from build123d import *

# Parameters (mm, degrees)
SKETCH1_R                = 85
BOSS_EXTRUDE1_DEPTH      = 3.175
SKETCH2_W                = 20
SKETCH2_H                = 18.160284919
SKETCH2_R                = 1.5
BOSS_EXTRUDE2_DEPTH      = 3.175
FILLET1_R                = 8
CIRPATTERN1_COUNT        = 3
FILLET1_OF_CIRPATTERN1_R = 8


with BuildPart() as part:
    # Sketch1 → Boss-Extrude1 (new body)
    with BuildSketch(Plane.XY):
        Circle(SKETCH1_R)
    extrude(amount=BOSS_EXTRUDE1_DEPTH)

    # Sketch2 → Boss-Extrude2 (add, through all)
    with BuildSketch(Plane.XY):
        with Locations((0, -93.48985754)):
            Rectangle(SKETCH2_W, SKETCH2_H)
        with Locations((0, -92.57)):
            Circle(SKETCH2_R, mode=Mode.SUBTRACT)
    boss_extrude2 = extrude(amount=BOSS_EXTRUDE2_DEPTH)

    # Fillet1
    fillet1_edges = [part.edges().sort_by_distance(p)[0] for p in [
        (-10, -84.409715081, 1.5875),
        (-10, -102.57, 1.5875),
        (10, -102.57, 1.5875),
        (10, -84.409715081, 1.5875),
    ]]
    fillet(fillet1_edges, radius=FILLET1_R)

    # CirPattern1: Boss-Extrude2 ×3 about axis
    cirpattern1_axis = Axis((0, 0, 0), (0, 0, 1))
    for i in range(1, CIRPATTERN1_COUNT):
        add(boss_extrude2.rotate(cirpattern1_axis, i * 360 / CIRPATTERN1_COUNT))

    # Fillet1 of CirPattern1
    fillet1_of_cirpattern1_edges = [part.edges().sort_by_distance(p)[0] for p in [
        (78.100957586, 33.544603502, 1.5875),
        (93.828225666, 42.624745962, 1.5875),
        (83.828225666, 59.945254038, 1.5875),
        (68.100957586, 50.865111578, 1.5875),
        (-68.100957586, 50.865111578, 1.5875),
        (-83.828225666, 59.945254038, 1.5875),
        (-93.828225666, 42.624745962, 1.5875),
        (-78.100957586, 33.544603502, 1.5875),
    ]]
    fillet(fillet1_of_cirpattern1_edges, radius=FILLET1_OF_CIRPATTERN1_R)


solid = part.part
Source: CAD feature listing. Evaluate the final solid. Frame: model axes, mm. Coordinates: 2 decimals unless noted, no trailing zeros. Loops run counter-clockwise (first coordinate to the right, second up) from the corner with the lowest first, then second, coordinate; pieces in that order, holes last. Notation, with made-up numbers: (-4.5, 15.5) - (12.5, 15.5) arc R22 cw to (12.5, 49.5) - close; hole circle Ø1 at (71.25, 19). An arc over 180 degrees is marked (long way). Return JSON: item names as keys, results as strings.
Q1. Contact query for flat-ended pins moving along their axis: P1, Ø1, axis at y = -92.5, z = 1.5, coming from the -X side; P2, Ø1.8, axis at x = 0, y = -92.57, coming from the -Z side. Output: stop coordinate, or through.
Results:
{"P1": "x = -10", "P2": "through"}
Q2. Material intervals for line 1 along Y through (x, z) = (0, 1.9); line 2 along X through (y, z) = (-92.57, 1.6); line 3 along X through (y, z) = (47, 2.8), sorted ascending.
Results:
{"line 1": "-102.57 to -94.07, -91.07 to 85", "line 2": "-10 to -1.5, 1.5 to 10", "line 3": "-90.77 to -81.49, -78.85 to 78.85, 81.49 to 90.77"}
Q3. Section C-C, the plane x = 53.5. Return loops of the section in (y, z) (3 decimals), plus the area to 3 significant figures.
Results:
{"outline": "(-66.051, 0) - (66.051, 0) - (66.051, 3.175) - (-66.051, 3.175) - close", "area": "419 mm2"}
Q4. Section B-B, the plane y = -17. Return loops of the section in (x, z) (3 decimals), plus the area to 3 significant figures.
Results:
{"outline": "(-83.283, 0) - (83.283, 0) - (83.283, 3.175) - (-83.283, 3.175) - close", "area": "529 mm2"}
Q5. Section A-A, the plane z = 1.5. Return loops of the section in (x, y) (3 decimals), plus the area to 3 significant figures.
Results:
{"outline": "(-89.828, 49.553) arc R8 ccw to (-86.9, 38.625) - (-84.017, 36.96) arc R8 cw to (-80.446, 27.449) arc R85 ccw to (-16.452, -83.393) arc R8 cw to (-10, -91.241) - (-10, -94.57) arc R8 ccw to (-2, -102.57) - (2, -102.57) arc R8 ccw to (10, -94.57) - (10, -91.241) arc R8 cw to (16.452, -83.393) arc R85 ccw to (80.446, 27.449) arc R8 cw to (84.017, 36.96) - (86.9, 38.625) arc R8 ccw to (89.828, 49.553) - (87.828, 53.017) arc R8 ccw to (76.9, 55.945) - (74.017, 54.281) arc R8 cw to (63.994, 55.944) arc R85 ccw to (-63.994, 55.944) arc R8 cw to (-74.017, 54.281) - (-76.9, 55.945) arc R8 ccw to (-87.828, 53.017) - close; hole circle Ø3 at (-80.168, 46.285); hole circle Ø3 at (0, -92.57); hole circle Ø3 at (80.168, 46.285)", "area": "23,700 mm2"}
Q6. Mould query, pull axis X, two halves, no side actions, for faces 1 (the cylindrical face through (-7.719, -100.164, 1.61)), 2 (the cylindrical face through (73.1, -43.375, 1.565)), 3 (the cylindrical face through (82.885, 56.767, 1.61)). Classes: released by +X, released by -X, zero draft, split by the parting line, or undercut.
Results:
{"face 1": "released by -X", "face 2": "released by +X", "face 3": "undercut"}
